For this review, take the finished solid that the model builds, in its own axes (mm). A direction names the side the tool comes from. Coordinates: 2 decimals unless noted, no trailing zeros. Loops run counter-clockwise (first coordinate to the right, second up) from the corner with the lowest first, then second, coordinate; pieces in that order, holes last. Notation, with made-up numbers: M 78.5,0 L 105.5,0 A6 ccw 105.5,5 Z; hole C 41.25,-6 d2. An arc over 180 degrees is marked long. Put each result on its own line as item: value.
```python
from build123d import *

# Parameters (mm, degrees)
ESTRUSIONE_ESTRUSIONE2_DEPTH                         = 20
FORO_LAMATO_PER_VITE_M4_A_TESTA_CILINDRI_D           = 4.5
FORO_LAMATO_PER_VITE_M4_A_TESTA_CILINDRI_DEPTH       = 15
FORO_LAMATO_PER_VITE_M4_A_TESTA_CILINDRI_CBORE_D     = 10
FORO_LAMATO_PER_VITE_M4_A_TESTA_CILINDRI_CBORE_DEPTH = 3.5
FORO_LAMATO_PER_VITE_M4_A_TESTA_CILINDRI_TIP         = 1.351936393
SCHIZZO6_R                                           = 7.5
TAGLIO_ESTRUSIONE1_DEPTH                             = 3
FORO_PER_VITE_M4_1_D                                 = 4
FORO_PER_VITE_M4_1_DEPTH                             = 9
FORO_PER_VITE_M4_1_TIP                               = 1.201721238


with BuildPart() as part:
    # Schizzo2 → Estrusione-Estrusione2 (new body)
    with BuildSketch(Plane(origin=(0, 0, 0), x_dir=(1, 0, 0), z_dir=(0, 1, 0))):
        Polygon((5, 30), (5, 10.303300859), (10.303300859, 5), (30, 5), (30, 0), (0, 0), (0, 30), align=None)
    extrude(amount=ESTRUSIONE_ESTRUSIONE2_DEPTH)

    # Foro lamato per Vite M4 a testa cilindrica piana-1
    with Locations(Plane(origin=(5, 0, 0), x_dir=(0, 0, -1), z_dir=(1, 0, 0))):
        with Locations((17.5, 10)):
            CounterBoreHole(FORO_LAMATO_PER_VITE_M4_A_TESTA_CILINDRI_D / 2, FORO_LAMATO_PER_VITE_M4_A_TESTA_CILINDRI_CBORE_D / 2, FORO_LAMATO_PER_VITE_M4_A_TESTA_CILINDRI_CBORE_DEPTH, depth=FORO_LAMATO_PER_VITE_M4_A_TESTA_CILINDRI_DEPTH)
            with Locations((0, 0, -(FORO_LAMATO_PER_VITE_M4_A_TESTA_CILINDRI_DEPTH + FORO_LAMATO_PER_VITE_M4_A_TESTA_CILINDRI_TIP / 2))):  # 118° drill point
                Cone(0, FORO_LAMATO_PER_VITE_M4_A_TESTA_CILINDRI_D / 2, FORO_LAMATO_PER_VITE_M4_A_TESTA_CILINDRI_TIP, mode=Mode.SUBTRACT)

    # Schizzo6 → Taglio-Estrusione1 (cut)
    with BuildSketch(Plane.XY):
        with Locations((20, 10)):
            Circle(SCHIZZO6_R)
    extrude(amount=-TAGLIO_ESTRUSIONE1_DEPTH, mode=Mode.SUBTRACT)

    # Foro per Vite M4-1
    with Locations(Plane(origin=(20, 10, 0), x_dir=(1, 0, 0), z_dir=(0, 0, 1))):
        with Locations((0, 0)):
            Hole(FORO_PER_VITE_M4_1_D / 2, depth=FORO_PER_VITE_M4_1_DEPTH)
            with Locations((0, 0, -(FORO_PER_VITE_M4_1_DEPTH + FORO_PER_VITE_M4_1_TIP / 2))):  # 118° drill point
                Cone(0, FORO_PER_VITE_M4_1_D / 2, FORO_PER_VITE_M4_1_TIP, mode=Mode.SUBTRACT)


solid = part.part
```
(1) Wall thickness on line 1 along Y through (x, z) = (4, -17.5); line 2 along Y through (x, z) = (0.5, -17.5); line 3 along X through (y, z) = (14, -21.25): over which ranges is each line inside the solid? List them lowest first. Write a range as [from, to].
Determined:
line 1: y = [0, 5], [15, 20]
line 2: y = [0, 7.75], [12.25, 20]
line 3: x = [0, 5]
(2) Add section C-C (x = 20). Write out the cut boundary in (y, z).
Determined:
outline: M 0,-5 L 8,-5 L 8,-3 L 2.5,-3 L 2.5,0 L 0,0 Z; M 12,-5 L 20,-5 L 20,0 L 17.5,0 L 17.5,-3 L 12,-3 Z
(3) Add section B-B (y = 10). Write out the cut boundary in (x, z), plus the area to 3 significant figures.
Determined:
outline: M 0,-30 L 5,-30 L 5,-22.5 L 1.5,-22.5 L 1.5,-19.75 L 0,-19.75 Z; M 0,-15.25 L 1.5,-15.25 L 1.5,-12.5 L 5,-12.5 L 5,-10.3 L 10.3,-5 L 18,-5 L 18,-3 L 12.5,-3 L 12.5,0 L 0,0 Z; M 22,-5 L 30,-5 L 30,0 L 27.5,0 L 27.5,-3 L 22,-3 Z
area: 194 mm^2
(4) Add section A-A (z = -17.5). Write out the cut boundary in (x, y).
Determined:
outline: M 0,0 L 5,0 L 5,5 L 1.5,5 L 1.5,7.75 L 0,7.75 Z; M 0,12.25 L 1.5,12.25 L 1.5,15 L 5,15 L 5,20 L 0,20 Z
(5) For pin 1 (1.5 mm diameter, centred on y = 7, z = -15, fed in from -X); pin 2 (12 mm diameter, centred on x = 20, y = 10, fed in from -Z); pin 3 (4.5 mm diameter, centred on x = 19, y = 8, fed in from +Z); pin 4 (8 mm diameter, centred on y = 7.5, z = -19.5, fed in from +X), all flat-tipped, find the tip position at first contact; note any pin that passes through.
Determined:
pin 1: stops at x = 0
pin 2: stops at z = -5
pin 3: stops at z = -3
pin 4: stops at x = 5
(6) Draft analysis for pull direction X (two halves, no side actions). For faces 1 (the cylindrical face through (21.474, 11.352, -4.014)), 2 (the flat face through (12, 10, 0)), 3 (the flat face through (30, 10, -3)), 4 (the cylindrical face through (14.048, 5.436, -1.479)), state which applies: +X half, -X half, draft (parallel to the pull), parting line (faces both ways), or undercut.
Determined:
face 1: undercut
face 2: draft
face 3: +X half
face 4: undercut
(7) Add section D-D (x = 14). Write out the cut boundary in (y, z).
Determined:
outline: M 0,-5 L 20,-5 L 20,0 L 14.5,0 L 14.5,-3 L 5.5,-3 L 5.5,0 L 0,0 Z
(8) Tool access review of faces 5 (the flat face through (2, 10, -30)), 6 (the flat face through (22, 8, -3)), 7 (the cylindrical face through (3.274, 14.957, -16.849)), 8 (the flat face through (5, 7.6, -22.5)), 9 (the flat face through (7, 0, -6)): name each direction out of +Z, -Z, +X, -X, +Y, -Y from which nothing blocks a thin tool from reaching the whole face with its end or side.
Determined:
face 5: -Z, +X, -X, +Y, -Y
face 6: +Z
face 7: +X
face 8: -Z, +X, +Y, -Y
face 9: +Z, -Z, +X, -X, -Y
